For this review, use the dimensioned drawing (mm, ordinates from the lowest corner) and the shaded views. A direction names the side the tool comes from. Round coordinates to 2 decimals unless told otherwise and drop trailing zeros. Loops run counter-clockwise (first coordinate to the right, second up) from the corner with the lowest first, then second, coordinate; pieces in that order, holes last. Notation, with made-up numbers: M 3.25,-9 L 54.25,-9 A18 cw 54.25,17 Z; hole C 14,53 d7. An arc over 180 degrees is marked long. One line per item, written item: value. Start each with the question number.
Item 1: For the marked faces 1 and 2, list the 3-axis set-ups (+Z, -Z, +X, -X, +Y, -Y) from which the entire face can be reached by the end or side of a thin tool; tool diameter is ignored.
Item 2: We need section B-B (z = 110). Write out the cut boundary in (x, y).
Item 3: We need section C-C (x = 154.5). Write out the cut boundary in (y, z) (3 decimals), then the cut area to 3 significant figures.
Item 4: Clearance check with flat-ended pins moving along their axes: pin 1 (23 mm diameter, centred on y = 23, z = 59, fed in from +X); pin 2 (5 mm diameter, centred on y = 47, z = 31.5, fed in from +X). State where each tip first meets the part, or that it passes through.
Item 5: We need section A-A (y = 10). Write out the cut boundary in (x, z) (3 decimals), then the cut area to 3 significant figures.
Item 6: For line 1 along X through (y, z) = (67, 55); line 2 along Z through (x, y) = (154.5, 6.5) (3 decimals); line 3 along X through (y, z) = (12.5, 30.5), list the stretches that pass through material, from the lowest coordinate up.
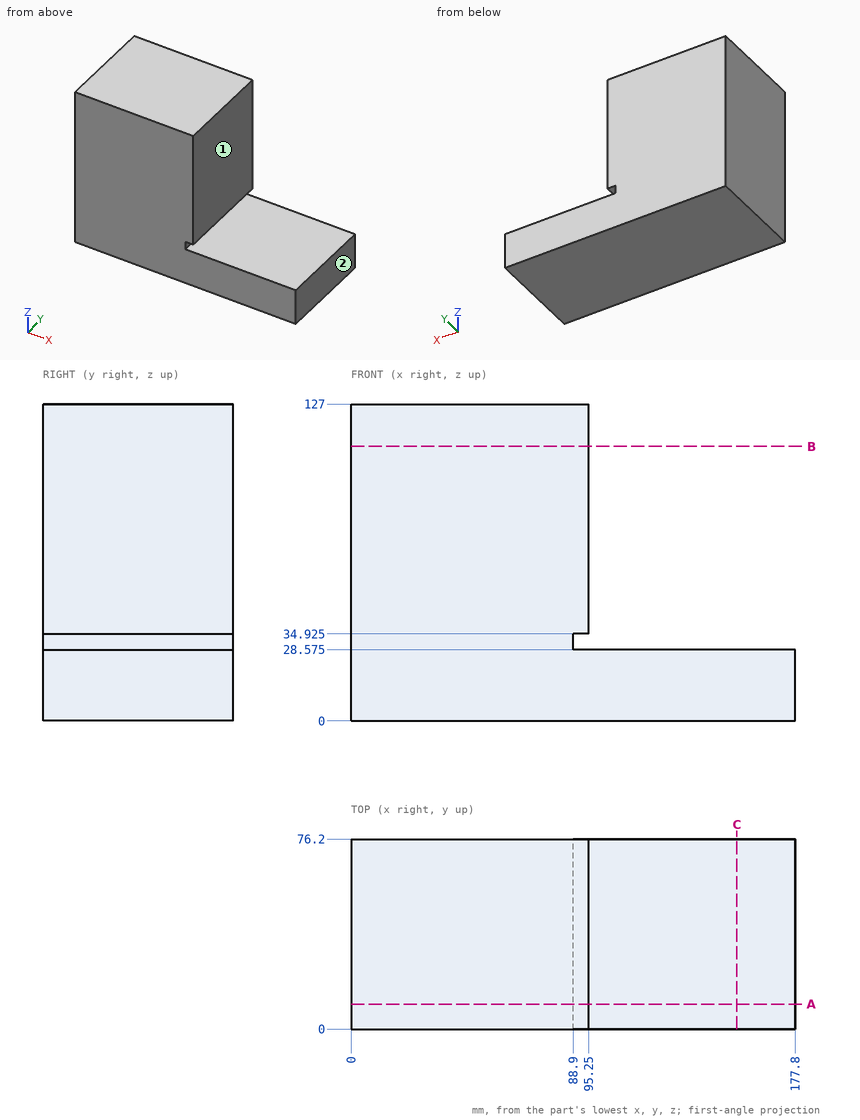
A:
1. face 1: +Z, +X, +Y, -Y
1. face 2: +Z, -Z, +X, +Y, -Y
2. outline: M 0,0 L 95.25,0 L 95.25,76.2 L 0,76.2 Z
3. outline: M 0,0 L 76.2,0 L 76.2,28.575 L 0,28.575 Z
3. area: 2,180 mm2
4. pin 1: x = 95.25
4. pin 2: x = 88.9
5. outline: M 0,0 L 177.8,0 L 177.8,28.575 L 88.9,28.575 L 88.9,34.925 L 95.25,34.925 L 95.25,127 L 0,127 Z
5. area: 14,400 mm2
6. line 1: 0 to 95.25
6. line 2: 0 to 28.575
6. line 3: 0 to 88.9
